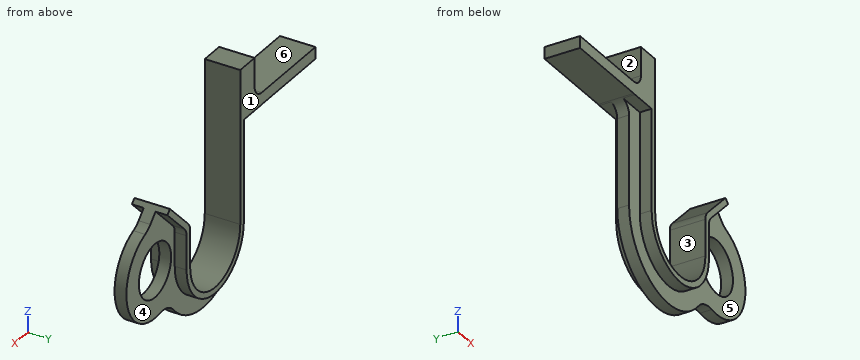
from build123d import *

# Parameters (mm, degrees)
BOSS_EXTRUDE1_DEPTH = 19.05
CUT_EXTRUDE3_START  = -6.35
CUT_EXTRUDE3_DEPTH  = 6.35
FILLET1_R           = 6.35
FILLET2_R           = 6.35
SKETCH4_W           = 6.35
SKETCH4_H           = 19.05
BOSS_EXTRUDE2_DEPTH = 63.5
SKETCH6_W           = 12.7
SKETCH6_H           = 19.05
BOSS_EXTRUDE3_DEPTH = 28.194
FILLET4_R           = 6.35
FILLET5_R           = 6.35
BOSS_EXTRUDE4_DEPTH = 6.35
FILLET6_R           = 12.7
FILLET7_R           = 12.7
SKETCH9_R           = 14.309078451
CUT_EXTRUDE5_DEPTH  = 122.979516723


with BuildPart() as part:
    # Sketch1 → Boss-Extrude1 (new body)
    with BuildSketch(Plane(origin=(0, 0, 0), x_dir=(1, 0, 0), z_dir=(0, 1, 0))):
        with BuildLine():
            Line((-22.225, 0), (-22.225, -82.55))
            Line((-22.225, -82.55), (-34.925, -82.55))
            Line((-34.925, -82.55), (-34.925, 0))
            ThreePointArc((-34.925, 0), (0, 34.925), (34.925, 0))
            Line((34.925, 0), (34.925, -16.964487758))
            Line((34.925, -16.964487758), (49.165768363, -31.205256121))
            Line((49.165768363, -31.205256121), (40.185512242, -40.185512242))
            Line((40.185512242, -40.185512242), (22.225, -22.225))
            Line((22.225, -22.225), (22.225, 0))
            ThreePointArc((22.225, 0), (0, 22.225), (-22.225, 0))
        make_face()
    extrude(amount=BOSS_EXTRUDE1_DEPTH)

    # Sketch3 → Cut-Extrude3 (cut)
    with BuildSketch(Plane(origin=(0, 19.05, 0), x_dir=(1, 0, 0), z_dir=(0, 1, 0)).offset(CUT_EXTRUDE3_START)):
        with BuildLine():
            Line((-34.925, 0), (-34.925, -82.55))
            Line((-34.925, -82.55), (-25.4, -82.55))
            Line((-25.4, -82.55), (-25.4, 0))
            ThreePointArc((-25.4, 0), (0, 25.4), (25.4, 0))
            Line((25.4, 0), (25.4, -20.909871939))
            Line((25.4, -20.909871939), (42.430576272, -37.940448212))
            Line((42.430576272, -37.940448212), (49.165768363, -31.205256121))
            Line((49.165768363, -31.205256121), (34.925, -16.964487758))
            Line((34.925, -16.964487758), (34.925, 0))
            ThreePointArc((34.925, 0), (0, 34.925), (-34.925, 0))
        make_face()
    cut_extrude3 = extrude(amount=CUT_EXTRUDE3_DEPTH, mode=Mode.SUBTRACT)

    # Mirror1: Cut-Extrude3 across plane
    add(cut_extrude3.mirror(Plane.ZX.offset(9.525)), mode=Mode.SUBTRACT)

    # Fillet1
    fillet1_edges = [part.edges().sort_by_distance(p)[0] for p in [
        (34.925, 9.525, 16.964487758),
        (25.4, 15.875, 20.909871939),
        (25.4, 3.175, 20.909871939),
    ]]
    fillet(fillet1_edges, radius=FILLET1_R)

    # Fillet2
    fillet2_edges = [part.edges().sort_by_distance(p)[0] for p in [
        (22.225, 9.525, 22.225),
    ]]
    fillet(fillet2_edges, radius=FILLET2_R)

    # Sketch4 → Boss-Extrude2 (add)
    with BuildSketch(Plane.ZY.offset(25.4)):
        with Locations((57.6072, 9.525)):
            Rectangle(SKETCH4_W, SKETCH4_H)
    extrude(amount=BOSS_EXTRUDE2_DEPTH)

    # Sketch6 → Boss-Extrude3 (add)
    with BuildSketch(Plane.XY.offset(82.55)):
        with Locations((-28.575, 9.525)):
            Rectangle(SKETCH6_W, SKETCH6_H)
    extrude(amount=-BOSS_EXTRUDE3_DEPTH)

    # Fillet4
    fillet4_edges = [part.edges().sort_by_distance(p)[0] for p in [
        (-34.925, 9.525, 60.7822),
    ]]
    fillet(fillet4_edges, radius=FILLET4_R)

    # Fillet5
    fillet5_edges = [part.edges().sort_by_distance(p)[0] for p in [
        (-34.925, 9.525, 54.4322),
    ]]
    fillet(fillet5_edges, radius=FILLET5_R)

    # Sketch8 → Boss-Extrude4 (add)
    with BuildSketch(Plane(origin=(0, 12.7, 0), x_dir=(1, 0, 0), z_dir=(0, 1, 0))):
        with BuildLine():
            Line((34.925, -14.334231637), (34.925, 0))
            ThreePointArc((34.925, 0), (33.953727024, 8.179244844), (31.093930783, 15.903556001))
            ThreePointArc((31.093930783, 15.903556001), (66.598964527, 2.503206576), (49.165768363, -31.205256121))
            Line((49.165768363, -31.205256121), (36.784871939, -18.824359697))
            ThreePointArc((36.784871939, -18.824359697), (35.408364969, -16.764271432), (34.925, -14.334231637))
        make_face()
    extrude(amount=-BOSS_EXTRUDE4_DEPTH)

    # Fillet6
    fillet6_edges = [part.edges().sort_by_distance(p)[0] for p in [
        (31.093930783, 9.525, -15.903556001),
    ]]
    fillet(fillet6_edges, radius=FILLET6_R)

    # Fillet7
    fillet7_edges = [part.edges().sort_by_distance(p)[0] for p in [
        (49.165768363, 9.525, 31.205256121),
    ]]
    fillet(fillet7_edges, radius=FILLET7_R)

    # Sketch9 → Cut-Extrude5 (cut, through all)
    with BuildSketch(Plane(origin=(0, 12.7, 0), x_dir=(1, 0, 0), z_dir=(0, 1, 0))):
        with Locations(Location((42.884078451, -6.594275404, 0), (0, 0, 270))):
            Circle(SKETCH9_R)
    extrude(amount=-CUT_EXTRUDE5_DEPTH, mode=Mode.SUBTRACT)


solid = part.part
Here's how the part is built. I have some questions about the finished solid (model axes, mm). Face numbers are marked on the shaded views. A direction names the side the tool comes from. Coordinates: 2 decimals unless noted, no trailing zeros. Write each loop counter-clockwise with the first axis right and the second up, starting at its lowest first coordinate (ties: lowest second). Pieces come first, ordered by that corner, then holes.
Item 1: I want a section at A-A on z = -9.5. Write out the boundary of the cut face in (x, y).
Item 2: On a 3-axis mill with a long thin cutter (end or side, diameter ignored), from which of +Z, -Z, +X, -X, +Y, -Y can I reach the whole of each face in a straight line? I mean the marked faces 4, 5 and 6. Say none if no direction works.
Item 3: If I drill on line 1 (X direction, y = 10.5, z = 13.5) (3 decimals); line 2 (X direction, y = 7.5, z = 3) (3 decimals); line 3 (X direction, y = 4.5, z = 6) (3 decimals), over which ranges is the centre line in solid material (lowest first)?
Item 4: If we mould it in two halves opening along X, with no side actions, what happens to the marked faces 1, 2 and 3? For each: +X half, -X half, draft (parallel to the pull), parting line (faces both ways), or undercut.
Item 5: I want a section at C-C on z = 5.5. Count the separate pieces of the cut face and the enclosed holes in it, and give its area (3 significant figures).
Item 6: I want a section at B-B on x = 0. Write out the boundary of the cut face in (y, z) (3 decimals).
Item 7: Will these pins go through, and if not, where does the flat tip stop? pin 1 (3 mm diameter, centred on y = 6, z = 38, fed in from -X) (3 decimals); pin 2 (10 mm diameter, centred on y = 6.5, z = -1, fed in from +X); pin 3 (1 mm diameter, centred on x = -15.5, y = 3, fed in from +Z).
Findings below:
1. outline: (-33.61, 6.35) - (-23.56, 6.35) - (-23.56, 0) - (-20.09, 0) - (-20.09, 19.05) - (-23.56, 19.05) - (-23.56, 12.7) - (-33.61, 12.7) - close; (20.09, 0) - (23.56, 0) - (23.56, 6.35) - (62.53, 6.35) - (62.53, 12.7) - (23.56, 12.7) - (23.56, 19.05) - (20.09, 19.05) - close
2. face 4: -Z, +Y
2. face 5: -Z, -Y
2. face 6: +Z, -X, +Y, -Y
3. line 1: x = -34.925 to -22.225, 22.225 to 30.352, 55.416 to 67.327
3. line 2: x = -34.925 to -22.225, 22.225 to 29.034, 56.734 to 68.028
3. line 3: x = -25.4 to -22.225, 22.225 to 25.4
4. face 1: draft
4. face 2: -X half
4. face 3: undercut
5. separate pieces: 3
5. enclosed holes: 0
5. area: 272 mm2
6. outline: (0, -25.4) - (6.35, -25.4) - (6.35, -34.925) - (12.7, -34.925) - (12.7, -25.4) - (19.05, -25.4) - (19.05, -22.225) - (0, -22.225) - close
7. pin 1: stops at x = -34.925
7. pin 2: stops at x = 68.15
7. pin 3: stops at z = -15.43
